from build123d import *

# Parameters (mm, degrees)
SKETCH1_W               = 278.13
SKETCH1_H               = 250.19
BOSS_EXTRUDE1_DEPTH     = 6.35
CUT_EXTRUDE2_DEPTH      = 375.154587704
CUT_EXTRUDE2_DEPTH_BACK = 375.154587704
SKETCH3_R               = 14.224
CUT_EXTRUDE4_DEPTH      = 375.154587704
CUT_EXTRUDE4_DEPTH_BACK = 375.154587704
SKETCH5_R               = 2.54
CUT_EXTRUDE5_DEPTH      = 375.154587704
CUT_EXTRUDE5_DEPTH_BACK = 375.154587704
SKETCH7_R               = 2.54


with BuildPart() as part:
    # Sketch1 → Boss-Extrude1 (new body)
    with BuildSketch(Plane.XY):
        with Locations((139.065, 125.095)):
            Rectangle(SKETCH1_W, SKETCH1_H)
    extrude(amount=BOSS_EXTRUDE1_DEPTH)

    # Sketch3 → Cut-Extrude2 (cut, two sides: drawn at the far end of the back side and taken through both)
    with BuildSketch(Plane.XY.offset(6.35).offset(-CUT_EXTRUDE2_DEPTH_BACK)):
        with Locations((63.5, 225.298)):
            Circle(SKETCH3_R)
        with Locations((215.9, 225.298)):
            Circle(SKETCH3_R)
        with Locations((34.544, 161.544)):
            Circle(SKETCH3_R)
        with Locations((242.824, 161.544)):
            Circle(SKETCH3_R)
        with Locations((49.53, 69.596)):
            Circle(SKETCH3_R)
        with Locations((227.33, 69.596)):
            Circle(SKETCH3_R)
    extrude(amount=CUT_EXTRUDE2_DEPTH + CUT_EXTRUDE2_DEPTH_BACK, mode=Mode.SUBTRACT)

    # Sketch5 → Cut-Extrude4 (cut, two sides: drawn at the far end of the back side and taken through both)
    with BuildSketch(Plane.XY.offset(6.35).offset(-CUT_EXTRUDE4_DEPTH_BACK)):
        with Locations((11.43, 228.346)):
            Circle(SKETCH5_R)
        with Locations((11.43, 202.946)):
            Circle(SKETCH5_R)
        with Locations((266.7, 202.946)):
            Circle(SKETCH5_R)
        with Locations((266.7, 228.346)):
            Circle(SKETCH5_R)
        with Locations((11.43, 115.062)):
            Circle(SKETCH5_R)
        with Locations((11.43, 89.662)):
            Circle(SKETCH5_R)
        with Locations((11.43, 64.262)):
            Circle(SKETCH5_R)
        with Locations((11.43, 38.862)):
            Circle(SKETCH5_R)
        with Locations((11.43, 13.462)):
            Circle(SKETCH5_R)
        with Locations((266.7, 115.062)):
            Circle(SKETCH5_R)
        with Locations((266.7, 89.662)):
            Circle(SKETCH5_R)
        with Locations((266.7, 64.262)):
            Circle(SKETCH5_R)
        with Locations((266.7, 38.862)):
            Circle(SKETCH5_R)
        with Locations((266.7, 13.462)):
            Circle(SKETCH5_R)
    extrude(amount=CUT_EXTRUDE4_DEPTH + CUT_EXTRUDE4_DEPTH_BACK, mode=Mode.SUBTRACT)

    # Sketch7 → Cut-Extrude5 (cut, two sides: drawn at the far end of the back side and taken through both)
    with BuildSketch(Plane.XY.offset(6.35).offset(-CUT_EXTRUDE5_DEPTH_BACK)):
        with Locations((16.51, 176.53)):
            Circle(SKETCH7_R)
        with Locations((16.51, 142.748)):
            Circle(SKETCH7_R)
        with Locations((52.324, 142.748)):
            Circle(SKETCH7_R)
        with Locations((52.324, 176.53)):
            Circle(SKETCH7_R)
        with Locations((225.806, 176.53)):
            Circle(SKETCH7_R)
        with Locations((261.62, 176.53)):
            Circle(SKETCH7_R)
        with Locations((225.806, 142.748)):
            Circle(SKETCH7_R)
        with Locations((261.62, 142.748)):
            Circle(SKETCH7_R)
    extrude(amount=CUT_EXTRUDE5_DEPTH + CUT_EXTRUDE5_DEPTH_BACK, mode=Mode.SUBTRACT)


solid = part.part
Design review of the part built by this model. Coordinates are the model's own, in mm. Coordinates: 2 decimals unless noted, no trailing zeros. Use a Markdown table: item, result.
(1) Draft analysis for pull direction Y (two halves, no side actions). For faces 1 (the cylindrical face through (62.67, 64.15, 3.13)), 2 (the flat face through (137, 0, 3)), 3 (the flat face through (0, 123, 3)), state which applies: released by +Y, released by -Y, zero draft, split by the parting line, or undercut.
Worked answers:
| item | result |
|---|---|
| face 1 | undercut |
| face 2 | released by -Y |
| face 3 | zero draft |
(2) Wall thickness on probe 1 along X at (y, z) = (176.53, 3); probe 2 along X at (y, z) = (236, 4); probe 3 along Y at (x, z) = (46, 0.5): over which ranges is each line inside the solid? List them lowest first.
Worked answers:
| item | result |
|---|---|
| probe 1 | x = 0 to 13.97, 19.05 to 49.78, 54.86 to 223.27, 228.35 to 259.08, 264.16 to 278.13 |
| probe 2 | x = 0 to 54.13, 72.87 to 206.53, 225.27 to 278.13 |
| probe 3 | y = 0 to 55.82, 83.38 to 153.11, 169.98 to 250.19 |
(3) Add section A-A (z = 5). Count the separate pieces of the cut face and the enclosed holes in it, then the cut area to 3 significant figures.
Worked answers:
| item | result |
|---|---|
| separate pieces | 1 |
| enclosed holes | 28 |
| area | 65,300 mm2 |
